Geometry check sheet. Reference: the model listing, model coordinates, mm. Face numbers are marked on the shaded views. A direction names the side the tool comes from. Round coordinates to 2 decimals unless told otherwise and drop trailing zeros. Write each loop counter-clockwise with the first axis right and the second up, starting at its lowest first coordinate (ties: lowest second). Pieces come first, ordered by that corner, then holes. Notation, with made-up numbers: M 50.5,27 L 101.5,27 A27 ccw 101.5,51 Z; hole C -20,-24 d11. An arc over 180 degrees is marked long. Answer in a Markdown table with one row per item. Add a question column.
from build123d import *

# Parameters (mm, degrees)
F0_R     = 1.75
F1_DEPTH = 7
F2_W     = 45
F2_H     = 54
F3_DEPTH = 19.5


with BuildPart() as f1:
    # F0 (on Top) → F1 (new body)
    with BuildSketch(Plane.XY):
        with BuildLine():
            ThreePointArc((19.5, -38.5), (21.62132, -37.62132), (22.5, -35.5))
            Line((22.5, -35.5), (22.5, 0))
            Line((22.5, 0), (22.5, 35.5))
            ThreePointArc((22.5, 35.5), (21.62132, 37.62132), (19.5, 38.5))
            Line((19.5, 38.5), (0, 38.5))
            Line((0, 38.5), (-19.5, 38.5))
            ThreePointArc((-19.5, 38.5), (-21.62132, 37.62132), (-22.5, 35.5))
            Line((-22.5, 35.5), (-22.5, 0))
            Line((-22.5, 0), (-22.5, -35.5))
            ThreePointArc((-22.5, -35.5), (-21.62132, -37.62132), (-19.5, -38.5))
            Line((-19.5, -38.5), (0, -38.5))
            Line((0, -38.5), (19.5, -38.5))
        make_face()
        with Locations((-18, -33.5)):
            Circle(F0_R, mode=Mode.SUBTRACT)
        with Locations((18, -33.5)):
            Circle(F0_R, mode=Mode.SUBTRACT)
        with Locations((-18, 33.5)):
            Circle(F0_R, mode=Mode.SUBTRACT)
        with Locations((18, 33.5)):
            Circle(F0_R, mode=Mode.SUBTRACT)
    extrude(amount=F1_DEPTH)

    # F2 (on face) → F3 (join)
    with BuildSketch(Plane.XY.offset(7)):
        Rectangle(F2_W, F2_H)
    extrude(amount=F3_DEPTH)


solid = f1.part
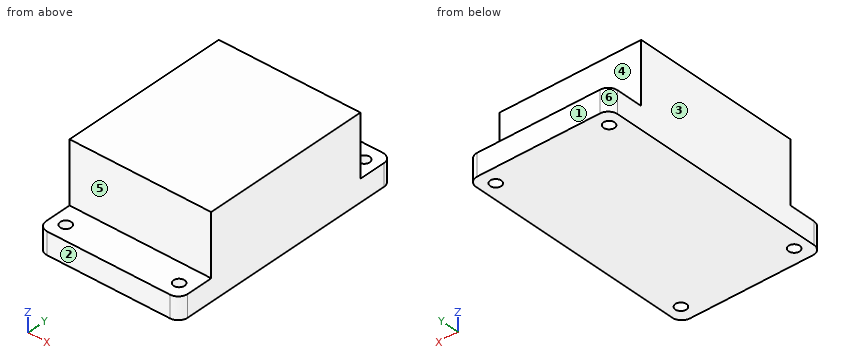
Item 1: Mould release check, pull along Y, two halves, no side actions. Record for the marked faces 1, 2 and 3: +Y half, -Y half, draft (parallel to the pull), parting line (faces both ways), or undercut.
Item 2: Access from +Z, -Z, +X, -X, +Y, -Y to the whole of each face (thin tool, end or side, straight path). Record for the marked faces 4, 5 and 6.
Item 3: Scan lines: probe 1 along Y at (x, z) = (-18, 4.25); probe 2 along Y at (x, z) = (-16, 15); probe 3 along Z at (x, y) = (13.5, -29.5). Record each from-to range of solid material in increasing order. Write a range as from..to.
Item 4: Section check A-A, the plane x = -18. Record the boundary of the cut face in (y, z), and give its area (3 significant figures).
Item 5: Section check D-D, the plane z = 9.25. Record the boundary of the cut face in (x, y).
Item 6: Gauge pin test, flat ends, axial feed: pin 1 Ø6 at (x, y) = (2, 31.5) entering from +Z; pin 2 Ø6 at (x, z) = (7, 17.5) entering from +Y; pin 3 Ø12 at (x, z) = (7.5, 15) entering from -Y; pin 4 Ø3 at (x, y) = (18, 33.5) entering from -Z. Record the tip position at first contact, or that the pin passes through.
Item 7: Section check C-C, the plane x = -13. Record the boundary of the cut face in (y, z).
Item 8: Section check B-B, the plane y = 33.5. Record the boundary of the cut face in (x, z).
Result sheet:
| question | item | result |
|---|---|---|
| 1 | face 1 | +Y half |
| 1 | face 2 | -Y half |
| 1 | face 3 | draft |
| 2 | face 4 | +Z, +X, -X, +Y |
| 2 | face 5 | +Z, +X, -X, -Y |
| 2 | face 6 | +Z, -Z, -X, +Y |
| 3 | probe 1 | y = -38.5..-35.25, -31.75..31.75, 35.25..38.5 |
| 3 | probe 2 | y = -27..27 |
| 3 | probe 3 | z = 0..7 |
| 4 | outline | M -38.5,0 L -35.25,0 L -35.25,7 L -38.5,7 Z; M -31.75,0 L 31.75,0 L 31.75,7 L 27,7 L 27,26.5 L -27,26.5 L -27,7 L -31.75,7 Z; M 35.25,0 L 38.5,0 L 38.5,7 L 35.25,7 Z |
| 4 | area | 1,540 mm^2 |
| 5 | outline | M -22.5,-27 L 22.5,-27 L 22.5,27 L -22.5,27 Z |
| 6 | pin 1 | stops at z = 7 |
| 6 | pin 2 | stops at y = 27 |
| 6 | pin 3 | stops at y = -27 |
| 6 | pin 4 | passes through |
| 7 | outline | M -38.5,0 L 38.5,0 L 38.5,7 L 27,7 L 27,26.5 L -27,26.5 L -27,7 L -38.5,7 Z |
| 8 | outline | M -22.5,0 L -19.75,0 L -19.75,7 L -22.5,7 Z; M -16.25,0 L 16.25,0 L 16.25,7 L -16.25,7 Z; M 19.75,0 L 22.5,0 L 22.5,7 L 19.75,7 Z |
